Build history of the part. All positions in model axes, mm. Face numbers are marked on the shaded views. Round coordinates to 2 decimals unless told otherwise and drop trailing zeros. Write each loop counter-clockwise with the first axis right and the second up, starting at its lowest first coordinate (ties: lowest second). Pieces come first, ordered by that corner, then holes. Notation, with made-up numbers: (86, 17.25) -> (103, 17.25) arc R31 ccw to (103, 41.25) -> close; hole circle Ø1 at (67.5, -4.5). An arc over 180 degrees is marked (long way). Return JSON: item names as keys, results as strings.
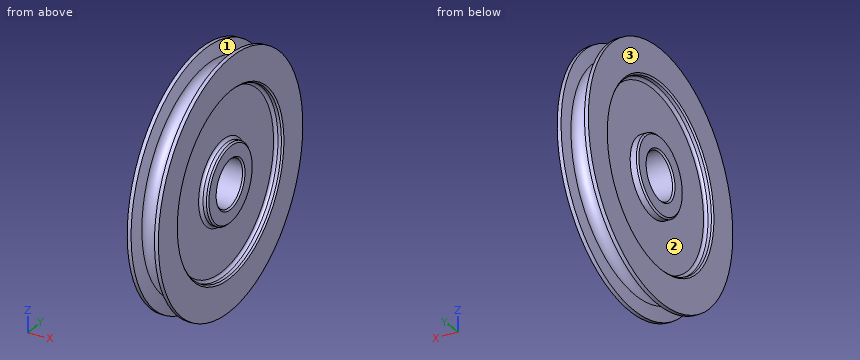
from build123d import *

# Parameters (mm, degrees)
F2_SIZE = 0.635
F3_R    = 1.143


with BuildPart() as f1:
    # F0 (on Front) → F1 (revolve)
    with BuildSketch(Plane.XZ):
        with BuildLine():
            Line((-0.370115592, 47.3796315491), (2.804884408, 47.3796315491))
            Line((2.804884408, 47.3796315491), (2.804884408, 26.4210365713))
            Line((2.804884408, 26.4210365713), (-0.370115592, 26.4246841986))
            Line((-0.370115592, 26.4246841986), (-0.370115592, 20.0444988011))
            Line((-0.370115592, 20.0444988011), (12.329884408, 20.0299082918))
            Line((12.329884408, 20.0299082918), (12.329884408, 26.3799082918))
            Line((12.329884408, 26.3799082918), (9.154884408, 26.3799082918))
            Line((9.154884408, 26.3799082918), (9.154884408, 47.3796315491))
            Line((9.154884408, 47.3796315491), (12.329884408, 47.3796315491))
            Line((12.329884408, 47.3796315491), (12.329884408, 61.3194988011))
            Line((12.329884408, 61.3194988011), (10.755084408, 61.3194988011))
            Line((10.755084408, 61.3194988011), (10.1112807135, 55.4913084055))
            ThreePointArc((10.1112807135, 55.4913084055), (6.1633464087, 51.9408858871), (2.2182688026, 55.4944823773))
            Line((2.2182688026, 55.4944823773), (1.204684408, 61.3194988011))
            Line((1.204684408, 61.3194988011), (-0.370115592, 61.3194988011))
            Line((-0.370115592, 61.3194988011), (-0.370115592, 47.3796315491))
        make_face()
    revolve(axis=Axis((7.6398788951, 0, 10.5194988011), (1, 0, 0)))

    # F2
    f2_edges = [f1.edges().sort_by_distance(p)[0] for p in [
        (12.329884, 0, -26.340634),
        (12.329884, 0, -5.340911),
        (12.329884, 0, 1.009089),
        (-0.370116, 0, 0.994499),
        (-0.370116, 0, -5.385687),
        (-0.370116, 0, -26.340634),
    ]]
    chamfer(f2_edges, length=F2_SIZE)

    # F3
    f3_edges = [f1.edges().sort_by_distance(p)[0] for p in [
        (2.804884, 0, -26.340634),
        (9.154884, 0, -26.340634),
        (9.154884, 0, -5.340911),
    ]]
    fillet(f3_edges, radius=F3_R)


solid = f1.part
Q1. Two-plate mould, pull along Z, no slides. Class the marked faces 1, 2 and 3: +Z half, -Z half, draft (parallel to the pull), parting line (faces both ways), or undercut.
Verdict:
{"face 1": "parting line", "face 2": "undercut", "face 3": "draft"}
Q2. Wall check: L1, parallel to Z at x = 0.85, y = 0; L2, parallel to Z at x = 11.35, y = 0; L3, parallel to Y at x = 11.25, z = 15. Give the ranges that are in metal, low to high.
Verdict:
{"L1": "z = -40.28 to -26.34, -5.38 to 1, 20.04 to 26.42, 47.38 to 61.32", "L2": "z = -40.28 to -26.34, -5.34 to 1.01, 20.03 to 26.38, 47.38 to 61.32", "L3": "y = -50.6 to -36.59, -15.21 to -8.39, 8.39 to 15.21, 36.59 to 50.6"}
Q3. Pin check, flat tips, straight feed: pin 1 Ø2 at (y, z) = (17.5, 20) entering from +X; pin 2 Ø1 at (x, z) = (3.5, 0) entering from -Y; pin 3 Ø5 at (x, z) = (2.5, 9) entering from +Y. Stop position of each tip, or through.
Verdict:
{"pin 1": "stops at x = 9.15", "pin 2": "stops at y = -41.7", "pin 3": "stops at y = 50.8"}
Q4. Saw through at A-A on x = 6.5. List the corners of the cut face in (y, z).
Verdict:
{"outline": "circle Ø82.87 at (0, 10.52); hole circle Ø19.03 at (0, 10.52)"}
